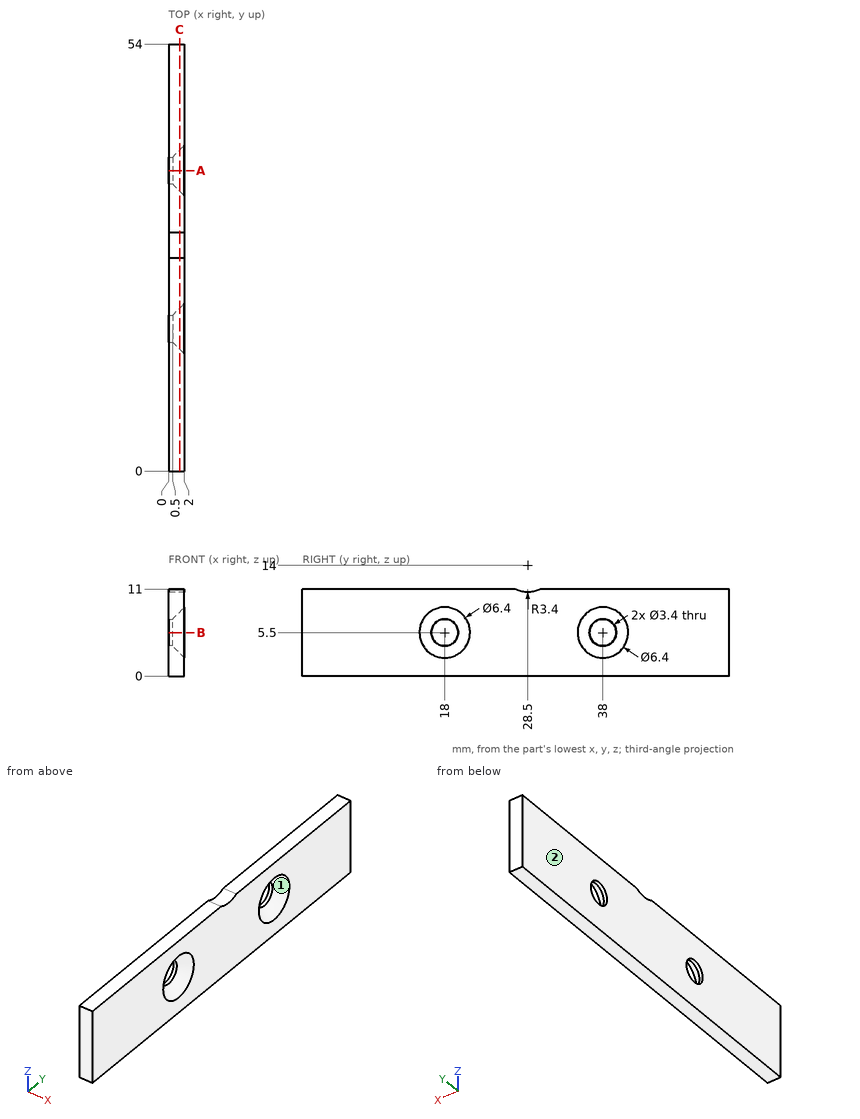
Source: three-view drawing plus pictorial views. Frame: mm from the lowest corner of the part. Coordinates: 2 decimals unless noted, no trailing zeros. Loops run counter-clockwise (first coordinate to the right, second up) from the corner with the lowest first, then second, coordinate; pieces in that order, holes last. Notation, with made-up numbers: (24, 21.5) - (70, 21.5) arc R17 ccw to (70, 50.5) - close; hole circle Ø5 at (-12.75, 66.25). An arc over 180 degrees is marked (long way). One line per item, written item: value. Start each with the question number.
1. Ray query, L1, parallel to Y at x = 0.2, z = 5.5; L2, parallel to Y at x = 0.45, z = 4.25; L3, parallel to Z at x = 0.3, y = 18. Return the intervals inside material, ascending.
2. Section A-A (y = 38). Return the cut outline in (x, z).
3. Contact query for flat-ended pins moving along their axis: P1, Ø4.5, axis at y = 18, z = 5.5, coming from the -X side; P2, Ø2.5, axis at y = 38, z = 5.5, coming from the -X side. Output: stop coordinate, or through.
4. Section C-C (x = 1.4). Return the cut outline in (y, z).
5. Mould query, pull axis Z, two halves, no side actions, for the marked faces 1 and 2. Classes: pulls with the +Z half, pulls with the -Z half, needs draft (parallel to the pull), parting line crosses it, or undercut.
6. Section B-B (z = 5.5). Return the cut outline in (x, y), and give its area (3 significant figures).
Verdict:
1. L1: y = 0 to 16.3, 19.7 to 36.3, 39.7 to 54
1. L2: y = 0 to 16.85, 19.15 to 36.85, 39.15 to 54
1. L3: z = 0 to 3.8, 7.2 to 11
2. outline: (0, 0) - (2, 0) - (2, 2.3) - (0.5, 3.8) - (0, 3.8) - close; (0, 7.2) - (0.5, 7.2) - (2, 8.7) - (2, 11) - (0, 11) - close
3. P1: stops at x = 0
3. P2: passes through
4. outline: (0, 0) - (54, 0) - (54, 11) - (30.1, 11) arc R3.4 cw to (26.9, 11) - (0, 11) - close; hole circle Ø5.2 at (18, 5.5); hole circle Ø5.2 at (38, 5.5)
5. face 1: undercut
5. face 2: needs draft
6. outline: (0, 0) - (2, 0) - (2, 14.8) - (0.5, 16.3) - (0, 16.3) - close; (0, 19.7) - (0.5, 19.7) - (2, 21.2) - (2, 34.8) - (0.5, 36.3) - (0, 36.3) - close; (0, 39.7) - (0.5, 39.7) - (2, 41.2) - (2, 54) - (0, 54) - close
6. area: 89.9 mm2
